Could you check a few things on this model? Use its own coordinates, in mm. Face numbers are marked on the shaded views. A direction names the side the tool comes from. Coordinates: 2 decimals unless noted, no trailing zeros. Order: outer loops, then holes, each group sorted by start corner. A loop starts at its lowest first (then second) coordinate and runs counter-clockwise, first axis right, second up. Notation, with made-up numbers: (26.5, 84) -> (33.5, 84) arc R22 cw to (33.5, 94) -> close; hole circle Ø5 at (67, 57.25). An arc over 180 degrees is marked (long way). Return JSON: item names as keys, results as strings. Group by question number.
from build123d import *

# Parameters (mm, degrees)
SKETCH2_W         = 31.75
SKETCH2_H         = 3.7846
SLOT_DEPTH        = 8.128
CIRPATTERN1_COUNT = 2
CIRPATTERN1_ANGLE = 90


# Read off the part's stored shape, not the designer's step: ThreadSchematic
with BuildPart() as part:
    # ThreadSchematic outline → ThreadSchematic (revolve)
    with BuildSketch(Plane.YX):
        with BuildLine():
            Line((0, 77.3938), (0, 0))
            ThreePointArc((0, 0), (10.548143245, 3.963989534), (15.875000001, 13.893800008))
            Line((15.875000001, 13.893800008), (9.525, 13.8938))
            Line((9.525, 13.8938), (9.525, 77.3938))
            Line((9.525, 77.3938), (0, 77.3938))
        make_face()
    revolve(axis=Axis((0, 0, 0), (1, 0, 0)))

    # Sketch2 → Slot (cut)
    with BuildSketch(Plane(origin=(0, 0, 0), x_dir=(0, 0, -1), z_dir=(1, 0, 0))):
        Rectangle(SKETCH2_W, SKETCH2_H)
    extrude(amount=SLOT_DEPTH, mode=Mode.SUBTRACT)

    # Sketch3 → Cross section 0
    with BuildSketch(Plane(origin=(0, 0, 0), x_dir=(0, 0, -1), z_dir=(1, 0, 0))):
        with BuildLine():
            Line((1.3081, -8.255), (-1.3081, -8.255))
            Line((-1.3081, -8.255), (-1.3081, 8.255))
            Line((-1.3081, 8.255), (1.3081, 8.255))
            Line((1.3081, 8.255), (1.3081, -8.255))
        make_face()
    # Sketch4 → Cross section 1
    with BuildSketch(Plane(origin=(10.0838, 0, 0), x_dir=(0, 0, -1), z_dir=(1, 0, 0))):
        with BuildLine():
            Line((0.65405, -0.65405), (-0.65405, -0.65405))
            Line((-0.65405, -0.65405), (-0.65405, 0.65405))
            Line((-0.65405, 0.65405), (0.65405, 0.65405))
            Line((0.65405, 0.65405), (0.65405, -0.65405))
        make_face()
    cross = loft(mode=Mode.SUBTRACT)

    # CirPattern1: Cross ×2 about axis
    cirpattern1_axis = Axis((0, 0, 0), (1, 0, 0))
    for i in range(1, CIRPATTERN1_COUNT):
        add(cross.rotate(cirpattern1_axis, i * CIRPATTERN1_ANGLE / (CIRPATTERN1_COUNT - 1)), mode=Mode.SUBTRACT)


solid = part.part
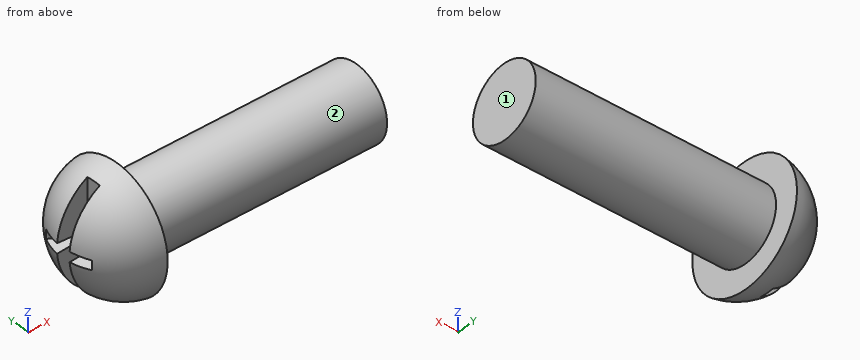
Q1. I'm going to push flat-ended pins straight in: pin 1 Ø1.1 at (y, z) = (0.5, -7.5) entering from -X; pin 2 Ø8 at (y, z) = (-9.5, 7) entering from -X; pin 3 Ø2 at (x, y) = (55, 9) entering from -Z; pin 4 Ø9.5 at (y, z) = (7.5, 7.5) entering from +X. Where does each tip first touch, or does it pass through?
Q2. On a 3-axis mill with a long thin cutter (end or side, diameter ignored), from which of +Z, -Z, +X, -X, +Y, -Y can I reach the whole of each face in a straight line? I mean the marked faces 1 and 2. Say none if no direction works.
Q3. I want a section at A-A on x = 22. Please give me the cut outline in (y, z) (3 decimals).
Q4. I want a section at C-C on y = 12. Please give me the cut outline in (x, z), and give its area (3 significant figures).
Q5. I want a section at B-B on y = -14. Please give me the cut outline in (x, z).
Q6. I need wall thicknesses on line 1 along X through (y, z) = (5, 13); line 2 along Z through (x, y) = (38, -0.5); line 3 along Y through (x, z) = (18, 2.5). Which ranges of each line are inside material? Lowest first, please. Write a range as from..to.
Response values:
{
 "1": {"pin 1": "stops at x = 8.13", "pin 2": "stops at x = 2.03", "pin 3": "stops at z = -5.17", "pin 4": "stops at x = 77.39"},
 "2": {"face 1": "+Z, -Z, +X, +Y, -Y", "face 2": "+X"},
 "3": {"outline": "circle Ø19.05 at (0, 0)"},
 "4": {"outline": "(13.89, -10.39) -> (13.89, 10.39) arc R10.61 ccw to start", "area": "132 mm²"},
 "5": {"outline": "(13.89, -7.48) -> (13.89, 7.48) arc R7.78 ccw to start"},
 "6": {"line 1": "x = 8.11..13.89", "line 2": "z = -9.51..9.51", "line 3": "y = -9.19..9.19"}
}
